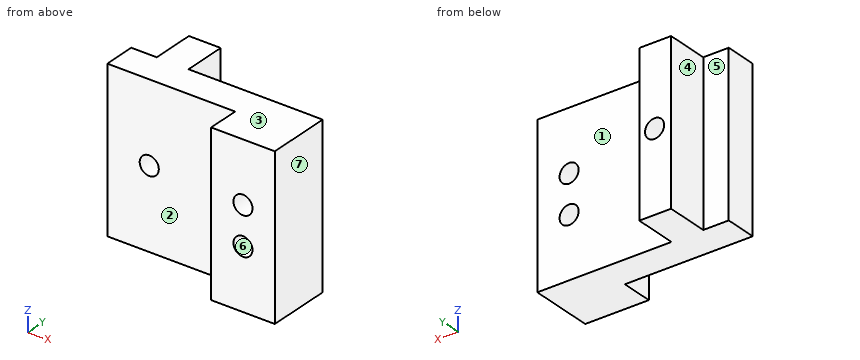
Autodesk Inventor part; units mm, degrees
ref_plane "YZ Plane" through (0, 0, 0) normal (1, 0, 0) x (0, 1, 0)
ref_plane "XZ Plane" through (0, 0, 0) normal (0, 1, 0) x (-1, 0, 0)
ref_plane "XY Plane" through (0, 0, 0) normal (0, 0, 1) x (1, 0, 0)
ref_plane "РабПлоскость1" through (-615.1898, 68.3314, 217.435) normal (0, 1, 0) x (-1, 0, 0)
sketch "Эскиз1" plane through (-615.1898, 68.3314, 217.435) normal (0, 1, 0) x (-1, 0, 0)
  circle A0 centre (-129, 47.5) radius 2
  circle A1 centre (-129, 41.5) radius 2
  line L0 (-129, 47.5) -> (-129, 41.5)
  line L1 (-134, 32) -> (-124, 32)
  line L2 (-124, 32) -> (-124, 57)
  line L3 (-124, 57) -> (-134, 57)
  line L4 (-134, 57) -> (-134, 32)
  line L5 (-134, 32) -> (-124, 57) construction
  line L6 (-124, 32) -> (-134, 57) construction
  point P0 (-615.1898, -217.435)
  point P1 (-129, 44.5)
  dimension "d0" = 25
  dimension "d1" = 10
extrude "Выдавливание1" add sketch "Эскиз1" along normal blind 5
sketch "Эскиз2" plane through (-615.1898, 73.3314, 217.435) normal (0, 1, 0) x (1, 0, 0)
  point P0 (615.1898, 217.435)
sketch "Эскиз3" plane through (-615.1898, 73.3314, 217.435) normal (0, 1, 0) x (1, 0, 0)
  point P0 (615.1898, 217.435)
sketch "Эскиз4" plane through (-615.1898, 73.3314, 217.435) normal (0, 1, 0) x (1, 0, 0)
  line L0 (134, -32) -> (124, -32)
  line L1 (134, -32) -> (103.9044, -32)
  line L2 (103.9044, -32) -> (103.9044, -57)
  line L3 (103.9044, -57) -> (134, -57)
  line L4 (134, -57) -> (134, -32)
  circle A0 centre (110.5, -44.5) radius 1.5
  point P0 (615.1898, 217.435)
extrude "Выдавливание2" add sketch "Эскиз4" along normal blind 5
sketch "Эскиз5" plane through (-615.1898, 78.3314, 217.435) normal (0, 1, 0) x (1, 0, 0)
  line L0 (124, -32) -> (103.9044, -32)
  line L1 (103.9044, -57) -> (124, -57)
  line L2 (107.9044, -32) -> (112.9044, -32)
  line L3 (112.9044, -32) -> (112.9044, -57)
  line L4 (112.9044, -57) -> (107.9044, -57)
  line L5 (107.9044, -57) -> (107.9044, -32)
  line L6 (103.9044, -32) -> (103.9044, -57)
  point P0 (615.1898, 217.435)
  point P1 (107.9044, -57)
  point P2 (112.9044, -32)
  dimension "d6" = 4
  dimension "d7" = 5
extrude "Выдавливание3" add sketch "Эскиз5" along normal up to surface (6.7181 mm away) contours L3 L1 L5 L0
sketch "Эскиз6" plane through (-507.2854, 85.0494, 274.435) normal (0, 1, 0) x (1, 0, 0)
  circle A0 centre (2.5956, 12.5) radius 1.5
  point P0 (507.2854, 274.435)
extrude "Выдавливание4" cut sketch "Эскиз6" against normal blind 17
sketch "Эскиз7" plane through (-615.1898, 68.3314, 217.435) normal (0, -1, 0) x (1, 0, 0)
  circle A0 centre (129, 41.5) radius 2
  circle A1 centre (129, 47.5) radius 2
  point P0 (615.1898, -217.435)
extrude "Выдавливание5" cut sketch "Эскиз7" against normal blind 14.5
sketch "Эскиз8" plane through (-615.1898, 78.3314, 217.435) normal (0, 1, 0) x (1, 0, 0)
  circle A0 centre (129, -41.5) radius 2
  circle A1 centre (129, -47.5) radius 2
  circle A2 centre (129, -41.5) radius 1.5
  circle A3 centre (129, -47.5) radius 1.5
  point P0 (615.1898, 217.435)
  dimension "d14" = 3
  dimension "d15" = 3
extrude "Выдавливание6" add sketch "Эскиз8" against normal up to surface (10 mm away)
sketch "Эскиз9" plane through (-507.2854, 85.0494, 274.435) normal (0, 1, 0) x (1, 0, 0)
  point P0 (507.2854, 274.435)
properties part number "крепление tcrt5000"
Verification items for the finished model (mm, model axes). Face numbers are marked on the shaded views. A direction names the side the tool comes from. Give positions to 0.01 mm unless a question says otherwise; leave off trailing zeros. Order: outer loops, then holes, each group sorted by start corner. A loop starts at its lowest first (then second) coordinate and runs counter-clockwise, first axis right, second up. Notation, with made-up numbers: (4, 4) -> (57, 4) arc R14 cw to (57, 15) -> close; hole circle Ø9 at (-25.5, 65). An arc over 180 degrees is marked (long way). Use a Markdown table: item, result.
1) Section check B-B, the plane y = 74. Record the boundary of the cut face in (x, z) (3 decimals), then the cut area to 3 significant figures.
Results:
| item | result |
|---|---|
| outline | (-511.285, 249.435) -> (-481.19, 249.435) -> (-481.19, 274.435) -> (-511.285, 274.435) -> close; hole circle Ø3 at (-504.69, 261.935); hole circle Ø3 at (-486.19, 258.935); hole circle Ø3 at (-486.19, 264.935) |
| area | 731 mm² |
2) Section check A-A, the plane z = 261.25. Record the boundary of the cut face in (x, y).
Results:
| item | result |
|---|---|
| outline | (-511.29, 73.33) -> (-506.02, 73.33) -> (-506.02, 85.05) -> (-507.29, 85.05) -> (-507.29, 78.33) -> (-511.29, 78.33) -> close; (-503.36, 73.33) -> (-491.19, 73.33) -> (-491.19, 68.33) -> (-481.19, 68.33) -> (-481.19, 78.33) -> (-502.29, 78.33) -> (-502.29, 85.05) -> (-503.36, 85.05) -> close |
3) Material ranges on probe 1 along Y at (x, z) = (-496, 255.75); probe 2 along Y at (x, z) = (-506.5, 259.25); probe 3 along Z at (x, y) = (-486, 72.25) (3 decimals), recorded low to high.
Results:
| item | result |
|---|---|
| probe 1 | 73.33 to 78.33 |
| probe 2 | 73.33 to 85.05 |
| probe 3 | 249.435 to 257.447, 260.423 to 263.447, 266.423 to 274.435 |
4) Section check D-D, the plane z = 253.75. Record the boundary of the cut face in (x, y).
Results:
| item | result |
|---|---|
| outline | (-511.29, 73.33) -> (-491.19, 73.33) -> (-491.19, 68.33) -> (-481.19, 68.33) -> (-481.19, 78.33) -> (-502.29, 78.33) -> (-502.29, 85.05) -> (-507.29, 85.05) -> (-507.29, 78.33) -> (-511.29, 78.33) -> close |
5) Mould release check, pull along X, two halves, no side actions. Record for the marked faces 4, 5, 6 and 7: pulls with the +X half, pulls with the -X half, needs draft (parallel to the pull), parting line crosses it, or undercut.
Results:
| item | result |
|---|---|
| face 4 | pulls with the -X half |
| face 5 | needs draft |
| face 6 | undercut |
| face 7 | pulls with the +X half |
6) Depth check by flat-ended pin: pin 1 Ø4 at (x, z) = (-497, 257.5) entering from -Y; pin 2 Ø6 at (x, z) = (-493.5, 268.5) entering from -Y; pin 3 Ø2 at (y, z) = (82.5, 268) entering from -X; pin 4 Ø5.5 at (y, z) = (70, 264.5) entering from -X. Enter the tip coordinate at first touch or a pass-through.
Results:
| item | result |
|---|---|
| pin 1 | y = 73.33 |
| pin 2 | y = 68.33 |
| pin 3 | x = -507.29 |
| pin 4 | x = -491.19 |
7) Section check C-C, the plane x = -490.5. Record the boundary of the cut face in (y, z) (3 decimals), then the cut area to 3 significant figures.
Results:
| item | result |
|---|---|
| outline | (68.331, 249.435) -> (78.331, 249.435) -> (78.331, 274.435) -> (68.331, 274.435) -> close |
| area | 250 mm² |
8) Tool access check on the marked faces 1, 2 and 3. Record the directions out of +Z, -Z, +X, -X, +Y, -Y that give a thin tool (end or side, any length) a straight path to the whole face; none if there is none.
Results:
| item | result |
|---|---|
| face 1 | +Z, -Z, +X, +Y |
| face 2 | +Z, -Z, -X, -Y |
| face 3 | +Z, +X, -X, +Y, -Y |
